from build123d import *

# Parameters (mm, degrees)
PAD014_DEPTH    = 14
POCKET017_DEPTH = 12
POCKET018_DEPTH = 6
SKETCH064_R     = 4
PAD015_DEPTH    = 3
SKETCH065_R     = 1.8
POCKET019_DEPTH = 5.001
SKETCH070_R     = 1.8
SKETCH070_W     = 10
SKETCH070_H     = 4
POCKET022_DEPTH = 2
SKETCH071_R     = 3.2
POCKET023_DEPTH = 2
FILLET003_R     = 2


with BuildPart() as part:
    # Sketch059 → Pad014 (new body)
    with BuildSketch(Plane.XY):
        with BuildLine():
            Line((61, 137.4), (79, 137.4))
            ThreePointArc((85, 131.4), (83.242641, 135.642641), (79, 137.4))
            Line((85, 131.4), (85, 79.644998))
            ThreePointArc((85, 79.644998), (82.64953, 80.948509), (80, 81.4))
            Line((80, 81.4), (55, 81.4))
            Line((55, 81.4), (55, 131.4))
            ThreePointArc((61, 137.4), (56.757359, 135.642641), (55, 131.4))
        make_face()
    extrude(amount=PAD014_DEPTH)

    # Sketch060 (on DatumPlane) → Pocket017 (cut)
    with BuildSketch(Plane.XY.offset(2)):
        with BuildLine():
            Line((61, 135.4), (79, 135.4))
            ThreePointArc((83, 131.4), (81.828427, 134.228427), (79, 135.4))
            Line((83, 131.4), (83, 83.4))
            Line((83, 83.4), (57, 83.4))
            Line((57, 83.4), (57, 131.4))
            ThreePointArc((61, 135.4), (58.171573, 134.228427), (57, 131.4))
        make_face()
    extrude(amount=POCKET017_DEPTH, mode=Mode.SUBTRACT)

    # Sketch063 (on Face5 of Pocket017) → Pocket018 (cut)
    with BuildSketch(Plane.XY.offset(14)):
        with BuildLine():
            Line((61, 137.4), (79, 137.4))
            ThreePointArc((85, 131.4), (83.242641, 135.642641), (79, 137.4))
            Line((85, 131.4), (85, 83.4))
            Line((85, 83.4), (55, 83.4))
            Line((55, 83.4), (55, 131.4))
            ThreePointArc((61, 137.4), (56.757359, 135.642641), (55, 131.4))
        make_face()
    extrude(amount=-POCKET018_DEPTH, mode=Mode.SUBTRACT)

    # Sketch064 (on Face20 of Pocket018) → Pad015 (join)
    with BuildSketch(Plane.XY.offset(2)):
        with Locations((70, 98.4)):
            Circle(SKETCH064_R)
    extrude(amount=PAD015_DEPTH)

    # Sketch065 (on Face22 of Pad015) → Pocket019 (cut, through all)
    with BuildSketch(Plane.XY.offset(5)):
        with Locations((70, 98.4)):
            Circle(SKETCH065_R)
    extrude(amount=-POCKET019_DEPTH, mode=Mode.SUBTRACT)

    # Sketch070 → Pocket022 (cut)
    with BuildSketch(Plane.XZ.offset(-81.4)):
        with Locations((63, 6)):
            Circle(SKETCH070_R)
        with Locations((75, 7)):
            Rectangle(SKETCH070_W, SKETCH070_H)
    extrude(amount=-POCKET022_DEPTH, mode=Mode.SUBTRACT)

    # Sketch071 (on Face2 of Pocket022) → Pocket023 (cut)
    with BuildSketch(Plane(origin=(0, 0, 0), x_dir=(1, 0, 0), z_dir=(0, 0, -1))):
        with Locations((70, -98.4)):
            Circle(SKETCH071_R)
    extrude(amount=-POCKET023_DEPTH, mode=Mode.SUBTRACT)

    # Fillet003
    fillet003_edges = [part.edges().sort_by_distance(p)[0] for p in [
        (66, 98.4, 2),
    ]]
    fillet(fillet003_edges, radius=FILLET003_R)


solid = part.part
CAD build for the part. Positions are in the model's coordinates, mm. A direction names the side the tool comes from. Round coordinates to 2 decimals unless told otherwise and drop trailing zeros. Write each loop counter-clockwise with the first axis right and the second up, starting at its lowest first coordinate (ties: lowest second). Pieces come first, ordered by that corner, then holes. Notation, with made-up numbers: (-36.5, -7) -> (-4.5, -7) arc R5 ccw to (-4.5, 0) -> close; hole circle Ø4 at (-2.5, 88). An arc over 180 degrees is marked (long way). Answer as a JSON object with one key per item and string values.
(1) Band-saw the part on B-B, the plane x = 63. List the corners of the cut face in (y, z).
Reported:
{"outline": "(81.4, 0) -> (137.4, 0) -> (137.4, 8) -> (135.4, 8) -> (135.4, 2) -> (83.4, 2) -> (83.4, 4.2) -> (81.4, 4.2) -> close; (81.4, 7.8) -> (83.4, 7.8) -> (83.4, 14) -> (81.4, 14) -> close"}
(2) Pin check, flat tips, straight feed: P1, Ø5, axis at x = 61, z = 3, coming from the -Y side; P2, Ø2, axis at x = 70, y = 98.4, coming from the +Z side; P3, Ø8, axis at x = 70.5, y = 114.5, coming from the +Z side; P4, Ø3, axis at x = 70, y = 97.5, coming from the -Z side. Stop position of each tip, or through.
Reported:
{"P1": "stops at y = 81.4", "P2": "passes through", "P3": "stops at z = 2", "P4": "stops at z = 2"}
(3) Which spindle directions (+Z, -Z, +X, -X, +Y, -Y) get a long thin tool onto all of the face, cutting with end or side? Do faces 1 (the face through (70, 82, 7)), 2 (the face through (70, 135.4, 5)), 3 (the face through (83.4, 114.5, 8)). Say none if no direction does.
Reported:
{"face 1": "-Y", "face 2": "+Z", "face 3": "+Z, +X, -X, +Y"}
(4) Band-saw the part on C-C, the plane z = 6. List the corners of the cut face in (x, y) (3 decimals), then the cut area to 3 significant figures.
Reported:
{"outline": "(55, 81.4) -> (61.2, 81.4) -> (61.2, 83.4) -> (57, 83.4) -> (57, 131.4) arc R4 cw to (61, 135.4) -> (79, 135.4) arc R4 cw to (83, 131.4) -> (83, 83.4) -> (80, 83.4) -> (80, 81.4) arc R8 cw to (85, 79.645) -> (85, 131.4) arc R6 ccw to (79, 137.4) -> (61, 137.4) arc R6 ccw to (55, 131.4) -> close; (64.8, 81.4) -> (70, 81.4) -> (70, 83.4) -> (64.8, 83.4) -> close", "area": "295 mm^2"}
(5) Probe probe 1 along X at (y, z) = (98.4, 3.85); probe 2 along Y at (x, z) = (70, 3.65); probe 3 along Z at (x, y) = (77, 83). List the from-to ranges inside material, lowest first. Write a range as [from, to].
Reported:
{"probe 1": "x = [55, 57], [65.99, 68.2], [71.8, 74.01], [83, 85]", "probe 2": "y = [81.4, 83.4], [94.37, 96.6], [100.2, 102.43], [135.4, 137.4]", "probe 3": "z = [0, 5], [9, 14]"}
(6) Band-saw the part on D-D, the plane y = 117.5. List the corners of the cut face in (x, z), then the cut area to 3 significant figures.
Reported:
{"outline": "(55, 0) -> (85, 0) -> (85, 8) -> (83, 8) -> (83, 2) -> (57, 2) -> (57, 8) -> (55, 8) -> close", "area": "84.0 mm^2"}
(7) Band-saw the part on A-A, the plane y = 98.4. List the corners of the cut face in (x, z).
Reported:
{"outline": "(55, 0) -> (66.8, 0) -> (66.8, 2) -> (68.2, 2) -> (68.2, 5) -> (66, 5) -> (66, 4) arc R2 cw to (64, 2) -> (57, 2) -> (57, 8) -> (55, 8) -> close; (71.8, 2) -> (73.2, 2) -> (73.2, 0) -> (85, 0) -> (85, 8) -> (83, 8) -> (83, 2) -> (76, 2) arc R2 cw to (74, 4) -> (74, 5) -> (71.8, 5) -> close"}
(8) Two-plate mould, pull along Y, no slides. Class faces 4 (the face through (70, 82, 14)), 5 (the face through (68, 81.4, 7)), 6 (the face through (70, 110, 2)), 7 (the face through (71.4, 99.8, 2)): +Y half, -Y half, draft (parallel to the pull), parting line (faces both ways), or undercut.
Reported:
{"face 4": "draft", "face 5": "-Y half", "face 6": "undercut", "face 7": "undercut"}
